```python
from build123d import *

# Parameters (mm, degrees)
SKETCH_1_W          = 25
SKETCH_1_H          = 47.2
EXTRUDE_1_DEPTH     = 14
CUT_EXTRUDE_1_DEPTH = 38.12088361
FILLET_1_R          = 15
SKETCH_3_W          = 24
SKETCH_3_H          = 13
SKETCH_3_R          = 0.5
CUT_EXTRUDE_2_DEPTH = 5
SKETCH_4_W          = 3.486393911
SKETCH_4_H          = 2.535559208
CUT_EXTRUDE_3_DEPTH = 5
SKETCH_5_R          = 0.679167645
EXTRUDE_2_DEPTH     = 50
FILLET_2_R          = 1


with BuildPart() as part:
    # 草圖1 → 填料-伸長1 (new body)
    with BuildSketch(Plane(origin=(0, 0, 0), x_dir=(1, 0, 0), z_dir=(0, 1, 0))):
        Rectangle(SKETCH_1_W, SKETCH_1_H)
    extrude(amount=EXTRUDE_1_DEPTH)

    # 草圖2 → 除料-伸長1 (cut, through all)
    with BuildSketch(Plane(origin=(12.5, 0, 0), x_dir=(0, 0, -1), z_dir=(1, 0, 0))):
        Polygon((-23.6, 10), (-3.6, 10), (11.6, 14), (-23.6, 14), align=None)
    extrude(amount=-CUT_EXTRUDE_1_DEPTH, mode=Mode.SUBTRACT)

    # 圓角1
    fillet_1_edges = [part.edges().sort_by_distance(p)[0] for p in [
        (0, 14, -11.6),
        (0, 10, 3.6),
    ]]
    fillet(fillet_1_edges, radius=FILLET_1_R)

    # 草圖3 → 除料-伸長2 (cut)
    with BuildSketch(Plane(origin=(0, 0, -23.6), x_dir=(-1, 0, 0), z_dir=(0, 0, -1))):
        with Locations((0, 7)):
            Rectangle(SKETCH_3_W, SKETCH_3_H)
        with Locations((-10.948606137, 12.643250156)):
            Circle(SKETCH_3_R, mode=Mode.SUBTRACT)
        with Locations((-7.948606137, 12.643250156)):
            Circle(SKETCH_3_R, mode=Mode.SUBTRACT)
        with Locations((-4.948606137, 12.643250156)):
            Circle(SKETCH_3_R, mode=Mode.SUBTRACT)
        with Locations((-1.948606137, 12.643250156)):
            Circle(SKETCH_3_R, mode=Mode.SUBTRACT)
        with Locations((1.051393863, 12.643250156)):
            Circle(SKETCH_3_R, mode=Mode.SUBTRACT)
        with Locations((4.051393863, 12.643250156)):
            Circle(SKETCH_3_R, mode=Mode.SUBTRACT)
        with Locations((7.051393863, 12.643250156)):
            Circle(SKETCH_3_R, mode=Mode.SUBTRACT)
        with Locations((10.051393863, 12.643250156)):
            Circle(SKETCH_3_R, mode=Mode.SUBTRACT)
        with Locations((-7.948606137, 9.843250156)):
            Circle(SKETCH_3_R, mode=Mode.SUBTRACT)
        with Locations((-4.948606137, 9.843250156)):
            Circle(SKETCH_3_R, mode=Mode.SUBTRACT)
        with Locations((-1.948606137, 9.843250156)):
            Circle(SKETCH_3_R, mode=Mode.SUBTRACT)
        with Locations((1.051393863, 9.843250156)):
            Circle(SKETCH_3_R, mode=Mode.SUBTRACT)
        with Locations((4.051393863, 9.843250156)):
            Circle(SKETCH_3_R, mode=Mode.SUBTRACT)
        with Locations((7.051393863, 9.843250156)):
            Circle(SKETCH_3_R, mode=Mode.SUBTRACT)
        with Locations((10.051393863, 9.843250156)):
            Circle(SKETCH_3_R, mode=Mode.SUBTRACT)
        with Locations((-7.948606137, 7.043250156)):
            Circle(SKETCH_3_R, mode=Mode.SUBTRACT)
        with Locations((-4.948606137, 7.043250156)):
            Circle(SKETCH_3_R, mode=Mode.SUBTRACT)
        with Locations((-1.948606137, 7.043250156)):
            Circle(SKETCH_3_R, mode=Mode.SUBTRACT)
        with Locations((1.051393863, 7.043250156)):
            Circle(SKETCH_3_R, mode=Mode.SUBTRACT)
        with Locations((4.051393863, 7.043250156)):
            Circle(SKETCH_3_R, mode=Mode.SUBTRACT)
        with Locations((7.051393863, 7.043250156)):
            Circle(SKETCH_3_R, mode=Mode.SUBTRACT)
        with Locations((10.051393863, 7.043250156)):
            Circle(SKETCH_3_R, mode=Mode.SUBTRACT)
        with Locations((-7.948606137, 4.243250156)):
            Circle(SKETCH_3_R, mode=Mode.SUBTRACT)
        with Locations((-4.948606137, 4.243250156)):
            Circle(SKETCH_3_R, mode=Mode.SUBTRACT)
        with Locations((-1.948606137, 4.243250156)):
            Circle(SKETCH_3_R, mode=Mode.SUBTRACT)
        with Locations((1.051393863, 4.243250156)):
            Circle(SKETCH_3_R, mode=Mode.SUBTRACT)
        with Locations((4.051393863, 4.243250156)):
            Circle(SKETCH_3_R, mode=Mode.SUBTRACT)
        with Locations((7.051393863, 4.243250156)):
            Circle(SKETCH_3_R, mode=Mode.SUBTRACT)
        with Locations((10.051393863, 4.243250156)):
            Circle(SKETCH_3_R, mode=Mode.SUBTRACT)
        with Locations((-7.948606137, 1.443250156)):
            Circle(SKETCH_3_R, mode=Mode.SUBTRACT)
        with Locations((-4.948606137, 1.443250156)):
            Circle(SKETCH_3_R, mode=Mode.SUBTRACT)
        with Locations((-1.948606137, 1.443250156)):
            Circle(SKETCH_3_R, mode=Mode.SUBTRACT)
        with Locations((1.051393863, 1.443250156)):
            Circle(SKETCH_3_R, mode=Mode.SUBTRACT)
        with Locations((4.051393863, 1.443250156)):
            Circle(SKETCH_3_R, mode=Mode.SUBTRACT)
        with Locations((7.051393863, 1.443250156)):
            Circle(SKETCH_3_R, mode=Mode.SUBTRACT)
        with Locations((10.051393863, 1.443250156)):
            Circle(SKETCH_3_R, mode=Mode.SUBTRACT)
        with Locations((-10.948606137, 9.843250156)):
            Circle(SKETCH_3_R, mode=Mode.SUBTRACT)
        with Locations((-10.948606137, 7.043250156)):
            Circle(SKETCH_3_R, mode=Mode.SUBTRACT)
        with Locations((-10.948606137, 4.243250156)):
            Circle(SKETCH_3_R, mode=Mode.SUBTRACT)
        with Locations((-10.948606137, 1.443250156)):
            Circle(SKETCH_3_R, mode=Mode.SUBTRACT)
    extrude(amount=-CUT_EXTRUDE_2_DEPTH, mode=Mode.SUBTRACT)

    # 草圖4 → 除料-伸長3 (cut)
    with BuildSketch(Plane.XY.offset(23.6)):
        with Locations((-9.968677216, 7.978706613)):
            Rectangle(SKETCH_4_W, SKETCH_4_H)
    extrude(amount=-CUT_EXTRUDE_3_DEPTH, mode=Mode.SUBTRACT)

    # 草圖5 → 填料-伸長2 (add)
    with BuildSketch(Plane.XY.offset(23.6)):
        with Locations(Location((0.875366181, 7.344816811, 0), (0, 0, 180))):
            Circle(SKETCH_5_R)
        with Locations(Location((3.875366181, 7.344816811, 0), (0, 0, 180))):
            Circle(SKETCH_5_R)
    extrude(amount=EXTRUDE_2_DEPTH)

    # 圓角2
    fillet_2_edges = [part.edges().sort_by_distance(p)[0] for p in [
        (-12.5, 14, -18.570324057),
        (-12.5, 10, 14.570324057),
        (12.5, 10, 14.570324057),
        (12.5, 14, -18.570324057),
        (12.5, 12, -4),
        (12.5, 13.876017123, -11.616040476),
        (-12.5, 12, -4),
        (-12.5, 13.876017123, -11.616040476),
        (12.5, 10.123982877, 3.616040476),
        (-12.5, 10.123982877, 3.616040476),
        (-12.5, 0, 0),
        (12.5, 0, 0),
    ]]
    fillet(fillet_2_edges, radius=FILLET_2_R)


solid = part.part
```
For this review, take the finished solid that the model builds, in its own axes (mm). A direction names the side the tool comes from. Give positions to 0.01 mm unless a question says otherwise; leave off trailing zeros. Loops run counter-clockwise (first coordinate to the right, second up) from the corner with the lowest first, then second, coordinate; pieces in that order, holes last. Notation, with made-up numbers: M 15,24 L 62,24 A20 cw 62,58 Z; hole C 45.25,57.5 d4. An arc over 180 degrees is marked long. One line per item, written item: value. Start each with the question number.
Q1. Add section A-A (z = 12). Give the boundary of the cut face in (x, y).
Q2. For L1, parallel to X at y = 7.5, z = 32.5; L2, parallel to Z at x = 0, y = 8.75; L3, parallel to Y at x = 1.5, z = 15, list the stretches that pass through material, from the lowest coordinate up.
Q3. Clearance check with flat-ended pins moving along their axes: pin 1 Ø5 at (x, z) = (-2.5, 58.5) entering from +Y; pin 2 Ø8 at (x, y) = (-3.5, 9.5) entering from +Z; pin 3 Ø6.5 at (x, y) = (-0.5, 6.5) entering from -Z; pin 4 Ø6 at (x, z) = (3, 63.5) entering from +Y. State where each tip first meets the part, or that it passes through.
Q4. Draft analysis for pull direction Y (two halves, no side actions). For faces 1 (the face through (-3.8, 0.2, -23.6)), 2 (the face through (-10, 8, 18.6)), 3 (the face through (-12, 7, -21)), 4 (the face through (-0.161, 10.127, 3.589)), state which applies: released by +Y, released by -Y, zero draft, split by the parting line, or undercut.
Q5. Add section B-B (z = 25). Give the boundary of the cut face in (x, y), and give its area (3 significant figures).
Q6. Machinability: for faces 5 (the face through (-8.225, 8, 21)), 6 (the face through (0, 10, 15)), 7 (the face through (0, 13.5, -21)), 8 (the face through (-12.5, 6, 0)), which of the approach directions +Z, -Z, +X, -X, +Y, -Y give a long, thin tool a straight path to every point of the face, cutting with its end or side? Answer none if there is none.
Reply:
1. outline: M -12.5,1 A1 ccw -11.5,0 L 11.5,0 A1 ccw 12.5,1 L 12.5,9 A1 ccw 11.5,10 L -11.5,10 A1 ccw -12.5,9 Z
2. L1: 0.21 to 1.54, 3.21 to 4.54
2. L2: -18.6 to 23.6
2. L3: 0 to 10
3. pin 1: through
3. pin 2: z = 23.6
3. pin 3: z = -23.6
3. pin 4: y = 8.02
4. face 1: zero draft
4. face 2: undercut
4. face 3: undercut
4. face 4: released by +Y
5. outline: C 0.88,7.34 d1.36; C 3.88,7.34 d1.36
5. area: 2.90 mm²
6. face 5: +Z
6. face 6: +Z, +X, -X, +Y
6. face 7: -Z
6. face 8: +Z, -Z, -X, +Y, -Y
